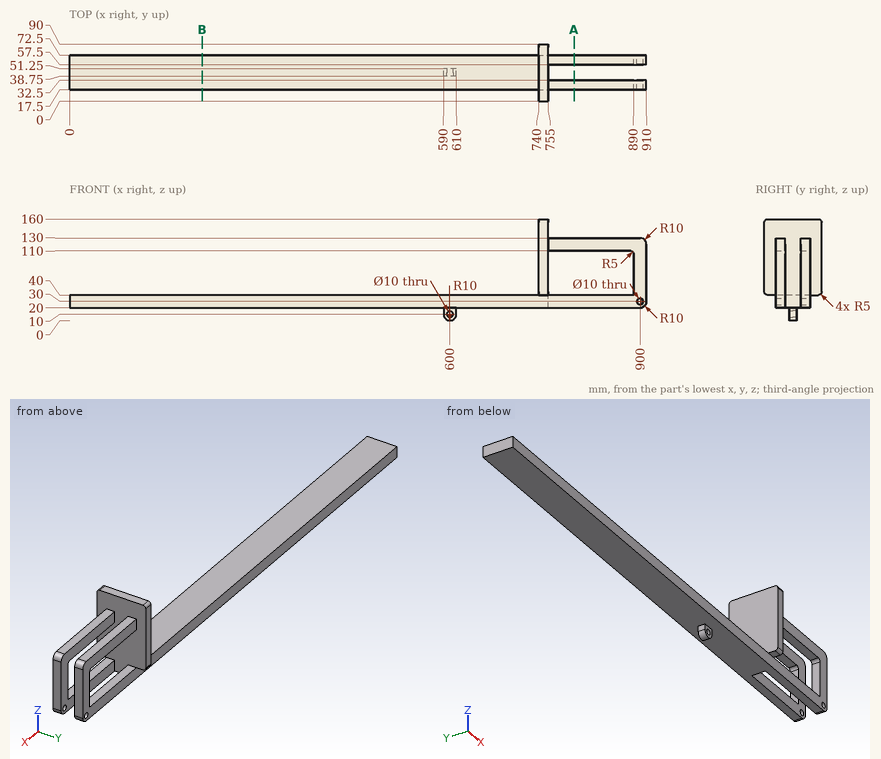
Answer from the drawing. Dimensions are ordinates in mm from the lowest x, y and z of the part. Round coordinates to 2 decimals unless told otherwise and drop trailing zeros. Loops run counter-clockwise (first coordinate to the right, second up) from the corner with the lowest first, then second, coordinate; pieces in that order, holes last.
Q1. Each of these flat-tipped pins is pushed along its axis until it touches: pin 1 (4.5 mm diameter, centred on x = 802.5, y = 62, fed in from +Z); pin 2 (6 mm diameter, centred on x = 326.5, y = 40, fed in from -Z); pin 3 (4 mm diameter, centred on x = 576, z = 34.5, fed in from +Y). Where does it stop, or does it pass through?
Q2. Section A-A on x = 796 is taken. Write down the section's boundary in (y, z).
Q3. Consider probe 1 along Z at (x, y) = (600, 48.75); probe 2 along Z at (x, y) = (813, 60.5); probe 3 along X at (y, z) = (62.5, 40.5). Determine where each line is inside the solid, lowest interval first.
Q4. Section B-B on x = 209 is taken. Write down the section's boundary in (y, z).
Output:
1. pin 1: stops at z = 130
1. pin 2: stops at z = 20
1. pin 3: stops at y = 72.5
2. outline: (17.5, 20) - (32.5, 20) - (32.5, 40) - (17.5, 40) - close; (17.5, 110) - (32.5, 110) - (32.5, 130) - (17.5, 130) - close; (57.5, 20) - (72.5, 20) - (72.5, 40) - (57.5, 40) - close; (57.5, 110) - (72.5, 110) - (72.5, 130) - (57.5, 130) - close
3. probe 1: z = 0 to 5, 15 to 40
3. probe 2: z = 20 to 40, 110 to 130
3. probe 3: x = 740 to 755, 890 to 910
4. outline: (17.5, 20) - (72.5, 20) - (72.5, 40) - (17.5, 40) - close
